Autodesk Inventor part; units mm, degrees
ref_plane "YZ Plane" through (0, 0, 0) normal (1, 0, 0) x (0, 1, 0)
ref_plane "XZ Plane" through (0, 0, 0) normal (0, 1, 0) x (-1, 0, 0)
ref_plane "XY Plane" through (0, 0, 0) normal (0, 0, 1) x (1, 0, 0)
sketch "Sketch1" plane through (0, 0, 0) normal (0, 0, 1) x (1, 0, 0)
  line L0 (0, 0) -> (80.8355, 0)
  line L1 (80.8355, 0) -> (80.8355, 152.4)
  line L2 (80.8355, 152.4) -> (0, 152.4)
  line L3 (0, 152.4) -> (0, 0)
  dimension "d82" = 80.8355
  dimension "d90" = 152.4
extrude "Extrusion1" add sketch "Sketch1" along normal blind 22.86
sketch "Sketch2" plane through (0, 0, 22.86) normal (0, 0, 1) x (1, 0, 0)
  line L0 (2.54, 2.54) -> (78.2955, 2.54)
  line L1 (78.2955, 2.54) -> (78.2955, 149.86)
  line L2 (78.2955, 149.86) -> (2.54, 149.86)
  line L3 (2.54, 149.86) -> (2.54, 2.54)
  line L4 (0, 152.4) -> (0, 0)
  line L5 (0, 0) -> (80.8355, 0)
  line L6 (80.8355, 0) -> (80.8355, 152.4)
  line L7 (80.8355, 152.4) -> (0, 152.4)
  line L8 (0, 152.4) -> (0, 0)
  line L9 (0, 0) -> (80.8355, 0)
  point P0 (80.8355, 76.2)
  point P1 (0, 76.2)
  point P2 (40.4177, 0)
  dimension "d83" = 152.4
  dimension "d85" = 80.8355
  dimension "d86" = 2.54
  dimension "d87" = 2.54
  dimension "d88" = 2.54
  dimension "d89" = 2.54
extrude "Extrusion2" cut sketch "Sketch2" against normal blind 19.05 contours L3 L2 L1 L0
sketch "Sketch6" plane through (0, 0, 3.81) normal (0, 0, 1) x (1, 0, 0)
  line L0 (5.1487, 87.2258) -> (75.6867, 87.2258) construction
  line L1 (75.6867, 87.2258) -> (75.6867, 3.2258) construction
  line L2 (75.6867, 3.2258) -> (5.1487, 3.2258) construction
  line L3 (5.1487, 3.2258) -> (5.1487, 87.2258) construction
  circle A0 centre (9.6205, 79.9318) radius 1.6 construction
  circle A1 centre (71.2409, 79.9318) radius 1.6 construction
  circle A2 centre (9.6205, 19.2258) radius 1.6 construction
  circle A3 centre (71.2409, 19.2258) radius 1.6 construction
  line L4 (2.54, 149.86) -> (78.2955, 149.86)
  line L5 (0, 0) -> (80.8355, 0)
  line L6 (78.2955, 2.54) -> (2.54, 2.54)
  circle A4 centre (9.6205, 79.9318) radius 4.445
  circle A5 centre (71.2409, 79.9318) radius 4.445
  circle A6 centre (9.6205, 19.2258) radius 4.445
  circle A7 centre (71.2409, 19.2258) radius 4.445
  point P0 (40.4177, 87.2258)
  point P1 (40.4177, 149.86)
  point P2 (3.175, 0)
  point P3 (77.6605, 0)
  point P4 (2.54, 2.54)
  point P5 (14.1287, 30.2258)
  point P6 (46.6867, 15.7258)
  point P7 (60.2637, 3.2258)
  point P8 (80.8355, 12.6941)
  dimension "d18" = 70.538
  dimension "d19" = 84
  dimension "d30" = 3.2
  dimension "d31" = 60.706
  dimension "d32" = 61.6204
  dimension "d33" = 16
  dimension "d34" = 4.4458
  dimension "d36" = 0.6858
  dimension "d37" = 27
  dimension "d38" = 8.98
  dimension "d39" = 12.5
  dimension "d40" = 29
  dimension "d41" = 15.423
  dimension "d69" = 8.89
  dimension "d70" = 8.89
  dimension "d71" = 8.89
  dimension "d72" = 8.89
extrude "Extrusion7" add sketch "Sketch6" along normal blind 2.54
sketch "Sketch15" plane through (9.6205, 79.9318, 6.35) normal (0, 0, 1) x (1, 0, 0)
  circle A0 centre (0, 0) radius 4.445
  circle A1 centre (61.6204, 0) radius 4.445
  circle A2 centre (61.6204, -60.706) radius 4.445
  circle A3 centre (0, -60.706) radius 4.445
  point P0 (-9.6205, -79.9318)
  point P1 (61.6204, -60.706)
  point P2 (0, -60.706)
hole "Hole3" at (9.6205, 79.9318, 6.35) at (71.2409, 79.9318, 6.35) at (71.2409, 19.2258, 6.35) at (9.6205, 19.2258, 6.35) direction (0, 0, -1) diameter 2.286 depth 6.35
sketch "Sketch16" plane through (0, 0, 3.81) normal (0, 0, 1) x (1, 0, 0)
  line L0 (10.6608, 147.32) -> (70.5655, 147.32)
  line L1 (70.5655, 147.32) -> (70.5655, 98.3851)
  line L2 (70.5655, 98.3851) -> (10.6608, 98.3851)
  line L3 (10.6608, 98.3851) -> (10.6608, 147.32)
  line L4 (2.54, 149.86) -> (78.2955, 149.86)
  point P0 (0, 0)
  dimension "d150" = 48.9349
  dimension "d151" = 59.9047
  dimension "d152" = 2.54
extrude "Extrusion8" cut sketch "Sketch16" against normal blind 25.4
sketch "Sketch17" plane through (2.54, 149.86, 22.86) normal (0, -1, 0) x (1, 0, 0)
  circle A0 centre (7.709, -8.0113) radius 1.27
  point P0 (-2.54, -22.86)
  dimension "d93" = 2.54
extrude "Extrusion9" cut sketch "Sketch17" along normal blind 25.4 and the other way blind 12.7 draft 60
sketch "Sketch18" plane through (10.6608, 98.3851, 3.81) normal (0, 1, 0) x (1, 0, 0)
  line L0 (59.9047, 0) -> (0, 0)
  line L1 (7.9345, 0) -> (11.287, 0)
  line L2 (11.287, 0) -> (11.287, 0.9229)
  line L3 (11.287, 0.9229) -> (7.9345, 0.9229)
  line L4 (7.9345, 0.9229) -> (7.9345, 0)
  line L5 (45.7582, 0) -> (49.8968, 0)
  line L6 (49.8968, 0) -> (49.8968, 0.9229)
  line L7 (49.8968, 0.9229) -> (45.7582, 0.9229)
  line L8 (45.7582, 0.9229) -> (45.7582, 0)
  point P0 (-10.6608, 3.81)
  point P1 (11.287, 0)
extrude "Extrusion10" cut sketch "Sketch18" against normal blind 2.54
sketch "Sketch19" plane through (0, 0, 3.81) normal (0, 0, 1) x (1, 0, 0)
  point P0 (0, 0)
sketch "Sketch23" plane through (0, 0, 0) normal (0, 0, -1) x (-1, 0, 0)
  line L0 (-84.6455, 152.4) -> (3.81, 152.4)
  line L1 (3.81, 152.4) -> (3.81, 0)
  line L2 (3.81, 0) -> (-84.6455, 0)
  line L3 (-84.6455, 0) -> (-84.6455, 152.4)
  line L4 (0, 0) -> (-80.8355, 0)
  line L5 (-80.8355, 152.4) -> (0, 152.4)
  line L6 (-80.8355, 0) -> (-80.8355, 152.4)
  line L7 (0, 152.4) -> (0, 0)
  point P0 (0, 152.4)
  dimension "d109" = 0
  dimension "d110" = 0
  dimension "d111" = 3.81
  dimension "d112" = 3.81
extrude "Extrusion12" add sketch "Sketch23" against normal blind 29.21 contours L0 L6 L2 L3 | L0 L1 L2 L7
sketch "Sketch24" plane through (84.6455, 0, 0) normal (1, 0, 0) x (0, 0, -1)
  line L0 (-29.21, 0) -> (-29.21, 152.4)
  line L1 (0, 152.4) -> (-29.21, 152.4)
  line L2 (0, 0) -> (-29.21, 0)
  point P0 (-26.035, 12.7)
  point P1 (-26.035, 139.7)
  dimension "d115" = 3.175
  dimension "d116" = 12.7
  dimension "d117" = 12.7
  dimension "d118" = 3.175
hole "Hole5" at (84.6455, 139.7, 26.035) at (84.6455, 12.7, 26.035) direction (-1, 0, 0) diameter 2.286 end through all
sketch "Sketch25" plane through (-3.81, 0, 0) normal (0, -1, 0) x (1, 0, 0)
  line L0 (3.81, 22.86) -> (84.6455, 22.86)
  line L1 (58.3565, 22.86) -> (69.7865, 22.86)
  line L2 (69.7865, 22.86) -> (69.7865, 7.62)
  line L3 (69.7865, 7.62) -> (58.3565, 7.62)
  line L4 (58.3565, 7.62) -> (58.3565, 22.86)
  line L5 (88.4555, 0) -> (88.4555, 29.21)
  point P0 (3.81, 0)
  point P1 (69.7865, 15.24)
  point P2 (64.0715, 22.86)
  point P3 (64.0715, 7.62)
  point P4 (44.2278, 22.86)
  dimension "d126" = 11.43
  dimension "d127" = 15.24
  dimension "d129" = 19.8438
extrude "Extrusion13" cut sketch "Sketch25" against normal up to surface (2.54 mm away)
sketch "Sketch26" plane through (-3.81, 0, 0) normal (0, -1, 0) x (1, 0, 0)
  line L0 (0, 29.21) -> (3.81, 29.21)
  line L1 (3.556, 29.21) -> (84.8995, 29.21)
  line L2 (84.8995, 29.21) -> (84.8995, 22.86)
  line L3 (84.8995, 22.86) -> (3.556, 22.86)
  line L4 (3.556, 22.86) -> (3.556, 29.21)
  line L5 (3.81, 22.86) -> (58.3565, 22.86)
  line L6 (3.81, 22.86) -> (3.81, 29.21)
  line L7 (84.6455, 22.86) -> (84.6455, 29.21)
  line L8 (3.81, 29.21) -> (84.6455, 29.21)
  line L9 (84.6455, 29.21) -> (84.6455, 22.86)
  line L10 (84.6455, 22.86) -> (3.81, 22.86)
  line L11 (3.81, 22.86) -> (3.81, 29.21)
  point P0 (3.81, 0)
  point P1 (84.8995, 26.035)
  dimension "d132" = 0
  dimension "d133" = 0.254
  dimension "d134" = 0.254
extrude "Extrusion14" cut sketch "Sketch26" against normal through all contours L0 L6 L3 L4 | L1 L2 L3 L7
sketch "Sketch27" plane through (-3.81, 0, 0) normal (0, -1, 0) x (1, 0, 0)
  line L0 (0, 29.21) -> (1.778, 29.21)
  line L1 (1.778, 29.21) -> (1.778, 0)
  line L2 (1.778, 0) -> (0, 0)
  line L3 (0, 0) -> (0, 29.21)
  line L4 (3.556, 22.86) -> (3.556, 29.21)
  line L5 (88.4555, 0) -> (88.4555, 29.21)
  line L6 (88.4555, 0) -> (0, 0)
  line L7 (88.4555, 29.21) -> (86.6775, 29.21)
  line L8 (86.6775, 29.21) -> (86.6775, 0)
  line L9 (86.6775, 0) -> (88.4555, 0)
  line L10 (88.4555, 0) -> (88.4555, 29.21)
  point P0 (3.81, 0)
  point P1 (0.889, 0)
  dimension "d137" = 1.778
  dimension "d138" = 1.778
  dimension "d139" = 0
extrude "Extrusion15" cut sketch "Sketch27" against normal through all
sketch "Sketch28" plane through (0, 0, 22.86) normal (0, 0, 1) x (1, 0, 0)
  line L0 (-0.254, 152.4) -> (81.0895, 152.4)
  line L1 (82.8675, 0) -> (-2.032, 0)
  line L2 (-0.254, 152.4) -> (81.0895, 152.4)
  line L3 (81.0895, 152.4) -> (81.0895, 0)
  line L4 (81.0895, 0) -> (-0.254, 0)
  line L5 (-0.254, 0) -> (-0.254, 152.4)
  line L6 (81.0895, 152.4) -> (81.0895, 0)
  line L7 (2.54, 149.86) -> (78.2955, 149.86)
  line L8 (78.2955, 149.86) -> (78.2955, 2.54)
  line L9 (2.54, 149.86) -> (78.2955, 149.86)
  line L10 (78.2955, 149.86) -> (78.2955, 2.54)
  line L11 (78.2955, 2.54) -> (2.54, 2.54)
  line L12 (2.54, 2.54) -> (2.54, 149.86)
  line L13 (54.5465, 2.54) -> (2.54, 2.54)
  line L14 (54.5465, 0) -> (54.5465, 2.54)
  line L15 (54.5465, 2.54) -> (54.5465, 0)
  line L16 (65.9765, 0) -> (65.9765, 2.54)
  line L17 (65.9765, 0) -> (65.9765, 2.54)
  line L18 (78.2955, 2.54) -> (2.54, 2.54)
  point P0 (0, 0)
  point P1 (-0.254, 0)
  dimension "d142" = 0
extrude "Extrusion16" add sketch "Sketch28" along normal blind 8.4667 contours L0 L3 L1 L16 L11 L8 L7 L12 L14 L5
sketch "Sketch29" plane through (0, 0, 29.21) normal (0, 0, 1) x (1, 0, 0)
  line L0 (-2.032, 152.4) -> (82.8675, 152.4)
  line L1 (-2.032, 152.4) -> (0, 152.4)
  line L2 (0, 152.4) -> (0, 0)
  line L3 (0, 0) -> (-2.032, 0)
  line L4 (-2.032, 0) -> (-2.032, 152.4)
  line L5 (82.8675, 0) -> (82.8675, 152.4)
  line L6 (81.0895, 0) -> (81.0895, 152.4)
  line L7 (82.8675, 152.4) -> (81.0895, 152.4)
  line L8 (81.0895, 152.4) -> (81.0895, 0)
  line L9 (81.0895, 0) -> (82.8675, 0)
  line L10 (82.8675, 0) -> (82.8675, 152.4)
extrude "Extrusion17" add sketch "Sketch29" along normal blind 8.4667
sketch "Sketch30" plane through (0, 0, 3.81) normal (0, 0, 1) x (1, 0, 0)
  line L0 (10.6608, 147.32) -> (70.5655, 147.32)
  line L1 (70.5655, 147.32) -> (70.5655, 98.3851)
  point P0 (0, 0)
  point P1 (53.6723, 150.7878)
  point P2 (57.4821, 140.1387)
  dimension "d154" = 3.4678
  dimension "d155" = 16.8932
sketch "Sketch31" plane through (0, 0, 0) normal (0, 0, -1) x (-1, 0, 0)
  line L0 (-70.5655, 147.32) -> (-10.6608, 147.32)
  line L1 (-70.5655, 98.3851) -> (-70.5655, 147.32)
  point P0 (0, 0)
  point P1 (-53.6723, 150.7878)
  dimension "d156" = 3.4678
  dimension "d157" = 16.8932
hole "Hole6" at (53.6723, 150.7878, 0) direction (0, 0, 1) diameter 2.286 depth 12.7
properties part number "Bottom_Shell"
Input: part model. Units: mm. Frame: model coordinates. A direction names the side the tool comes from. Coordinates: 2 decimals unless noted, no trailing zeros. Order: outer loops, then holes, each group sorted by start corner. A loop starts at its lowest first (then second) coordinate and runs counter-clockwise, first axis right, second up. Notation, with made-up numbers: M -34.75,-31.5 L -12.75,-31.5 A24 ccw -12.75,3.5 Z; hole C 81.25,16 d8. An arc over 180 degrees is marked long. Answer as CSV lines item,"result".
1. First-contact query: P1, Ø3.5, axis at x = 71.24, y = 79.93, coming from the +Z side; P2, Ø3, axis at x = 62, y = 99, coming from the +Z side; P3, Ø1.1, axis at y = 12.5, z = 26.5, coming from the -X side; P4, Ø1.4, axis at x = 71.24, y = 19.23, coming from the -Z side. Flat tips, straight axial feed; report the tip coordinate or a pass-through.
Reported:
P1,"z = 6.35"
P2,"z = 3.81"
P3,"x = -0.25"
P4,"through"
2. Section A-A (y = 121.5). Return the cut outline in (x, z), then the cut area to 3 significant figures.
Reported:
outline,"M -2.03,0 L 10.66,0 L 10.66,3.81 L 2.54,3.81 L 2.54,31.33 L 0,31.33 L 0,37.68 L -2.03,37.68 Z; M 70.57,0 L 82.87,0 L 82.87,37.68 L 81.09,37.68 L 81.09,31.33 L 78.3,31.33 L 78.3,3.81 L 70.57,3.81 Z"
area,"371 mm2"
3. Access query for faces 1 (the flat face through (40, 147.32, 2)), 2 (the flat face through (41, 2.54, 17)), 3 (the flat face through (0, 77, 34)). Directions: +Z, -Z, +X, -X, +Y, -Y. A direction counts if a zero-diameter tool reaches every point of the face in a straight line with its end or side. Return the directions, or none.
Reported:
face 1,"+Z, -Z"
face 2,"+Z"
face 3,"+Z, +Y, -Y"
4. Section C-C (y = 41). Return the cut outline in (x, z).
Reported:
outline,"M -2.03,0 L 82.87,0 L 82.87,37.68 L 81.09,37.68 L 81.09,31.33 L 78.3,31.33 L 78.3,3.81 L 2.54,3.81 L 2.54,31.33 L 0,31.33 L 0,37.68 L -2.03,37.68 Z"
5. Pull-direction query (Z, two-part tool) for faces 4 (the conical face through (10.048, 150.019, 13.317)), 5 (the flat face through (40, 61, 3.81)), 6 (the cylindrical face through (11.67, 23.17, 5.06)); classes: released by +Z, released by -Z, zero draft, split by the parting line, or undercut.
Reported:
face 4,"undercut"
face 5,"released by +Z"
face 6,"zero draft"
6. Material intervals for line 1 (X direction, y = 115, z = 32); line 2 (Y direction, x = 15.5, z = 28); line 3 (X direction, y = 26, z = 22.5), sorted ascending. Write a range as from..to.
Reported:
line 1,"-2.03..0, 81.09..82.87"
line 2,"0..2.54, 149.86..152.4"
line 3,"-2.03..2.54, 78.3..82.87"
7. Section D-D (x = 32.5). Return the cut outline in (y, z).
Reported:
outline,"M 0,0 L 98.39,0 L 98.39,3.81 L 2.54,3.81 L 2.54,31.33 L 0,31.33 Z; M 147.32,0 L 152.4,0 L 152.4,31.33 L 149.86,31.33 L 149.86,3.81 L 147.32,3.81 Z"
8. Section B-B (x = 62). Return the cut outline in (y, z), then the cut area to 3 significant figures.
Reported:
outline,"M 0,0 L 98.39,0 L 98.39,3.81 L 2.54,3.81 L 2.54,7.62 L 0,7.62 Z; M 147.32,0 L 152.4,0 L 152.4,31.33 L 149.86,31.33 L 149.86,3.81 L 147.32,3.81 Z"
area,"474 mm2"
